Here's how the part is built. I have some questions about the finished solid (model axes, mm). A direction names the side the tool comes from. Give positions to 0.01 mm unless a question says otherwise; leave off trailing zeros. Loops run counter-clockwise (first coordinate to the right, second up) from the corner with the lowest first, then second, coordinate; pieces in that order, holes last. Notation, with made-up numbers: (84, 84.5) -> (130, 84.5) arc R25 ccw to (130, 111.5) -> close; hole circle Ø7 at (55, 35.25). An arc over 180 degrees is marked (long way). Answer in a Markdown table with one row per item. Add a question column.
Item 1: Which directions (+Z, -Z, +X, -X, +Y, -Y) give clear straight access to the entire face, cutting with the end or side of a thin tool? Please do faces 1 (the face through (-219.97, 5.45, 0.05)), 2 (the face through (-208.685, 6.76, 23.465)), 3 (the face through (-216, 4, 0)), 4 (the face through (-208.726, 6.76, -23.095)).
Item 2: If we section it at D-D (z = 28.5): Write out the boundary of the cut face in (x, y), then the cut area to 3 significant figures.
Item 3: If we section it at B-B (y = 4.75): Write out the boundary of the cut face in (x, z).
Item 4: If we section it at C-C (z = 0): Write out the boundary of the cut face in (x, y), then the cut area to 3 significant figures.
Item 5: For P1, Ø3, axis at y = 6.5, z = -1.5, coming from the +X side; P2, Ø4, axis at y = 6, z = -18.5, coming from the +X side; P3, Ø4, axis at x = -214.5, y = 1, coming from the +Z side, each with a flat end and sliding along its axis, tell me the tip position at first contact or that it passes through.
Item 6: We'd pull the mould along X, two halves only. Please class faces 5 (the face through (-211.837, 2.864, -37.353)), 6 (the face through (-212.75, 3.04, 19.33)), 7 (the face through (-213, 7.5, -1)): released by +X, released by -X, zero draft, split by the parting line, or undercut.
Item 7: If we section it at A-A (x = -205.75): Write out the boundary of the cut face in (y, z), then the cut area to 3 significant figures.
Item 8: If I drill on line 1 (Z direction, x = -211.5, y = 7); line 2 (Y direction, x = -213.25, z = -24); line 3 (X direction, y = 6.5, z = -19), over which ranges is the centre line in solid material (lowest first)?
```python
from build123d import *

# Parameters (mm, degrees)
BOSS_EXTRUDE1_DEPTH        = 7.5
CUT_EXTRUDE1_DEPTH         = 1.5
SKETCH4_R                  = 3.5
CUT_EXTRUDE3_DEPTH         = 2.5
SKETCH5_R                  = 2.05
CUT_EXTRUDE4_DEPTH         = 41.774005634
F_3_1_3_1_DIAMETER_HOLE1_D = 3.1


with BuildPart() as part:
    # Sketch1 → Boss-Extrude1 (new body)
    with BuildSketch(Plane(origin=(0, 0, 0), x_dir=(1, 0, 0), z_dir=(0, 1, 0))):
        with BuildLine():
            Line((-219.119725045, 38.636719531), (-204.34760875, 36.031996866))
            ThreePointArc((-204.34760875, 36.031996866), (-207.5, 0), (-204.34760875, -36.031996866))
            Line((-204.34760875, -36.031996866), (-219.119725045, -38.636719531))
            ThreePointArc((-219.119725045, -38.636719531), (-222.5, 0), (-219.119725045, 38.636719531))
        make_face()
    extrude(amount=BOSS_EXTRUDE1_DEPTH)

    # Sketch2 → Cut-Extrude1 (cut)
    with BuildSketch(Plane(origin=(0, 7.5, 0), x_dir=(1, 0, 0), z_dir=(0, 1, 0))):
        with BuildLine():
            Line((-206.809628133, 36.46611731), (-216.657705663, 38.202599087))
            ThreePointArc((-216.657705663, 38.202599087), (-218.670303662, 24.151569236), (-219.772609758, 10))
            Line((-219.772609758, 10), (-209.761769634, 10))
            ThreePointArc((-209.761769634, 10), (-208.70564487, 23.279901188), (-206.809628133, 36.46611731))
        make_face()
        with BuildLine():
            Line((-209.761769634, -10), (-219.772609758, -10))
            ThreePointArc((-219.772609758, -10), (-218.670303662, -24.151569236), (-216.657705663, -38.202599087))
            Line((-216.657705663, -38.202599087), (-206.809628133, -36.46611731))
            ThreePointArc((-206.809628133, -36.46611731), (-208.70564487, -23.279901188), (-209.761769634, -10))
        make_face()
    extrude(amount=-CUT_EXTRUDE1_DEPTH, mode=Mode.SUBTRACT)

    # Sketch4 → Cut-Extrude3 (cut)
    with BuildSketch(Plane(origin=(-215, 0, 0), x_dir=(0, 0, -1), z_dir=(1, 0, 0))):
        with Locations((0, 7.5)):
            Circle(SKETCH4_R)
    extrude(amount=-CUT_EXTRUDE3_DEPTH, mode=Mode.SUBTRACT)

    # Sketch5 → Cut-Extrude4 (cut, through all)
    with BuildSketch(Plane(origin=(-215, 0, 0), x_dir=(0, 0, -1), z_dir=(1, 0, 0))):
        with Locations((0, 7.5)):
            Circle(SKETCH5_R)
    extrude(amount=-CUT_EXTRUDE4_DEPTH, mode=Mode.SUBTRACT)

    # Ø3.1 (3.1) Diameter Hole1 (through all)
    with Locations(Plane(origin=(0, 0, 0), x_dir=(-1, 0, 0), z_dir=(0, -1, 0))):
        with Locations((214.18186009, -18.738484691), (214.18186009, 18.738484691)):
            Hole(F_3_1_3_1_DIAMETER_HOLE1_D / 2)


solid = part.part
```
Recorded:
| question | item | result |
|---|---|---|
| 1 | face 1 | -X, +Y |
| 1 | face 2 | +Z, +Y |
| 1 | face 3 | +Y |
| 1 | face 4 | -Z, +Y |
| 2 | outline | (-220.67, 0) -> (-205.53, 0) -> (-205.53, 7.5) -> (-208.06, 7.5) -> (-208.06, 6) -> (-218.15, 6) -> (-218.15, 7.5) -> (-220.67, 7.5) -> close |
| 2 | area | 98.4 mm^2 |
| 3 | outline | (-219.12, -38.64) -> (-204.35, -36.03) arc R207.5 cw to (-204.35, 36.03) -> (-219.12, 38.64) arc R222.5 ccw to start; hole (-217.5, -2.17) -> (-215, -2.17) -> (-215, 2.17) -> (-217.5, 2.17) -> close; hole circle Ø3.1 at (-214.18, -18.74); hole circle Ø3.1 at (-214.18, 18.74) |
| 4 | outline | (-222.5, 0) -> (-207.5, 0) -> (-207.5, 7.5) -> (-215, 7.5) -> (-215, 4) -> (-217.5, 4) -> (-217.5, 5.45) -> (-222.5, 5.45) -> close |
| 4 | area | 93.5 mm^2 |
| 5 | P1 | stops at x = -207.48 |
| 5 | P2 | stops at x = -206.48 |
| 5 | P3 | stops at z = 38.17 |
| 6 | face 5 | released by +X |
| 6 | face 6 | undercut |
| 6 | face 7 | zero draft |
| 7 | outline | (0, -36.28) -> (7.5, -36.28) -> (7.5, -26.89) -> (0, -26.89) -> close; (0, 26.89) -> (7.5, 26.89) -> (7.5, 36.28) -> (0, 36.28) -> close |
| 7 | area | 141 mm^2 |
| 8 | line 1 | z = -10 to 10 |
| 8 | line 2 | y = 0 to 6 |
| 8 | line 3 | x = -221.69 to -219.18, -209.14 to -206.63 |
